```python
from build123d import *

# Parameters (mm, degrees)
F0_R     = 6
F0_R_2   = 1.65
F1_DEPTH = 3
F2_R     = 6
F3_DEPTH = 5.5
F5_DEPTH = 3
F6_R     = 0.5
F7_R     = 2.4
F8_DEPTH = 5


with BuildPart() as f1:
    # F0 (on Top) → F1 (new body)
    with BuildSketch(Plane.XY):
        Circle(F0_R)
        with Locations((-3.175, 0)):
            Circle(F0_R_2, mode=Mode.SUBTRACT)
        with Locations((3.175, 0)):
            Circle(F0_R_2, mode=Mode.SUBTRACT)
    extrude(amount=F1_DEPTH)

    # F2 (on face) → F3 (join)
    with BuildSketch(Plane(origin=(0, 0, 0), x_dir=(1, 0, 0), z_dir=(0, 0, -1))):
        Circle(F2_R)
    extrude(amount=F3_DEPTH)

    # F4 (on face) → F5 (cut)
    with BuildSketch(Plane.XY.offset(3)):
        with BuildLine():
            ThreePointArc((3.968627, 4.5), (0, 6), (-3.968627, 4.5))
            Line((-3.968627, 4.5), (-1.968627, 4.5))
            Line((-1.968627, 4.5), (-1.968627, 2.5))
            Line((-1.968627, 2.5), (1.968627, 2.5))
            Line((1.968627, 2.5), (1.968627, 4.5))
            Line((1.968627, 4.5), (3.968627, 4.5))
        make_face()
    extrude(amount=-F5_DEPTH, mode=Mode.SUBTRACT)

    # F6
    f6_edges = [f1.edges().sort_by_distance(p)[0] for p in [
        (-3.968627, 4.5, 1.5),
        (-1.968627, 4.5, 1.5),
        (1.968627, 2.5, 1.5),
        (1.968627, 4.5, 1.5),
        (3.968627, 4.5, 1.5),
        (-1.968627, 2.5, 1.5),
    ]]
    fillet(f6_edges, radius=F6_R)

    # F7 (on face) → F8 (cut)
    with BuildSketch(Plane(origin=(0, 0, -5.5), x_dir=(1, 0, 0), z_dir=(0, 0, -1))):
        Circle(F7_R)
    extrude(amount=-F8_DEPTH, mode=Mode.SUBTRACT)


solid = f1.part
```
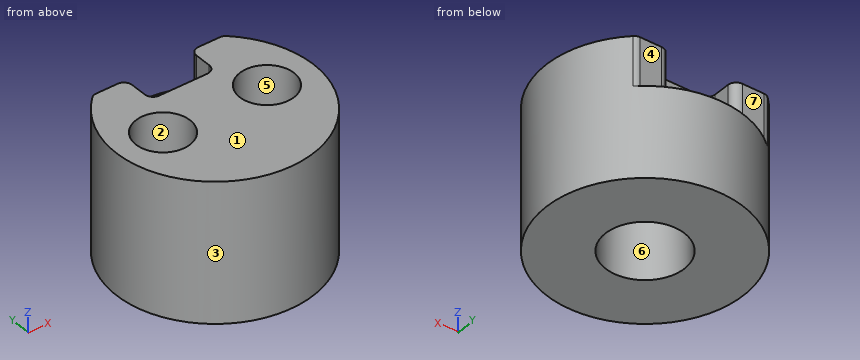
Check sheet for the modelled part. Datum: model origin and axes. Units: mm. Face numbers are marked on the shaded views. A direction names the side the tool comes from. Round coordinates to 2 decimals unless told otherwise and drop trailing zeros. Order: outer loops, then holes, each group sorted by start corner. A loop starts at its lowest first (then second) coordinate and runs counter-clockwise, first axis right, second up. Notation, with made-up numbers: (55.5, 53.5) - (94.5, 53.5) arc R20 ccw to (94.5, 70.5) - close; hole circle Ø10 at (82, 48.25). An arc over 180 degrees is marked (long way). Answer as CSV lines item,"result". Start each with the question number.
1) Section check B-B (z = 1.5). Record the cut outline in (x, y) (3 decimals), then the cut area to 3 significant figures.
2) Draft check along Y on the marked faces 1, 2, 3 and 4. Enter one of: +Y half, -Y half, draft (parallel to the pull), parting line (faces both ways), or undercut.
3) Scan lines: probe 1 along Y at (x, z) = (0, -2.1); probe 2 along Z at (x, y) = (2.5, -1.25). Record each from-to range of solid material in increasing order.
4) Depth check by flat-ended pin: pin 1 (4 mm diameter, centred on x = -4.5, z = 2, fed in from +Y); pin 2 (1.4 mm diameter, centred on x = -1, y = 0, fed in from -Z); pin 3 (1.6 mm diameter, centred on x = 3.5, y = -0.5, fed in from +Z). Enter the tip coordinate at first touch or a pass-through.
5) Tool access check on the marked faces 5, 6 and 7. Record the directions out of +Z, -Z, +X, -X, +Y, -Y that give a thin tool (end or side, any length) a straight path to the whole face; none if there is none.
6) Section check C-C (y = 0). Record the cut outline in (x, z) (3 decimals).
7) Section check A-A (x = 0). Record the cut outline in (y, z).
8) Section check D-D (z = -2). Record the cut outline in (x, y).
Determined:
1,outline,"(-4.118, 4.364) arc R6 ccw (long way) to (4.118, 4.364) arc R0.5 ccw to (3.775, 4.5) - (2.469, 4.5) arc R0.5 ccw to (1.969, 4) - (1.969, 3) arc R0.5 cw to (1.469, 2.5) - (-1.469, 2.5) arc R0.5 cw to (-1.969, 3) - (-1.969, 4) arc R0.5 ccw to (-2.469, 4.5) - (-3.775, 4.5) arc R0.5 ccw to start; hole circle Ø3.3 at (-3.175, 0); hole circle Ø3.3 at (3.175, 0)"
1,area,"79.9 mm^2"
2,face 1,"draft"
2,face 2,"undercut"
2,face 3,"parting line"
2,face 4,"+Y half"
3,probe 1,"-6 to -2.4, 2.4 to 6"
3,probe 2,"-5.5 to 0"
4,pin 1,"y = 4.5"
4,pin 2,"z = -0.5"
4,pin 3,"z = 0"
5,face 5,"+Z"
5,face 6,"-Z"
5,face 7,"+Z, +X, -X, +Y"
6,outline,"(-6, -5.5) - (-2.4, -5.5) - (-2.4, -0.5) - (2.4, -0.5) - (2.4, -5.5) - (6, -5.5) - (6, 3) - (4.825, 3) - (4.825, 0) - (1.525, 0) - (1.525, 3) - (-1.525, 3) - (-1.525, 0) - (-4.825, 0) - (-4.825, 3) - (-6, 3) - close"
7,outline,"(-6, -5.5) - (-2.4, -5.5) - (-2.4, -0.5) - (2.4, -0.5) - (2.4, -5.5) - (6, -5.5) - (6, 0) - (2.5, 0) - (2.5, 3) - (-6, 3) - close"
8,outline,"circle Ø12 at (0, 0); hole circle Ø4.8 at (0, 0)"
